Design review of the part built by this model. Coordinates are the model's own, in mm. Face numbers are marked on the shaded views. A direction names the side the tool comes from. Coordinates: 2 decimals unless noted, no trailing zeros. Order: outer loops, then holes, each group sorted by start corner. A loop starts at its lowest first (then second) coordinate and runs counter-clockwise, first axis right, second up. Notation, with made-up numbers: (77.25, 34.25) -> (124.25, 34.25) arc R12 ccw to (124.25, 50.25) -> close; hole circle Ø8 at (31.25, 17.5). An arc over 180 degrees is marked (long way). Write item = value, one per line.
```python
from build123d import *

# Parameters (mm, degrees)
SALIENTE_EXTRUIR1_DEPTH = 8
CROQUIS2_R              = 4.875
SALIENTE_EXTRUIR2_DEPTH = 28
MATRIZL1_COUNT          = 2
MATRIZL1_PITCH          = 25
MATRIZL1_COUNT_DIR2     = 2
MATRIZL1_PITCH_DIR2     = 25
CROQUIS3_R              = 2.65
CORTAR_EXTRUIR1_DEPTH   = 5.3
CROQUIS4_W              = 9.313425885
CROQUIS4_H              = 1.82271115
CROQUIS4_H_2            = 1.039944003
CROQUIS4_W_2            = 1.041549228
CROQUIS4_H_3            = 6.922662644
CROQUIS4_H_4            = 1.224371708
CORTAR_EXTRUIR2_DEPTH   = 2.5


with BuildPart() as part:
    # Croquis1 → Saliente-Extruir1 (new body)
    with BuildSketch(Plane(origin=(0, 0, 0), x_dir=(1, 0, 0), z_dir=(0, 1, 0))):
        with BuildLine():
            Line((-14.479225386, 25.911355575), (15.520774614, 25.911355575))
            ThreePointArc((15.520774614, 25.911355575), (22.591842426, 22.982423386), (25.520774614, 15.911355575))
            Line((25.520774614, 15.911355575), (25.520774614, -14.088644425))
            ThreePointArc((25.520774614, -14.088644425), (22.591842426, -21.159712237), (15.520774614, -24.088644425))
            Line((15.520774614, -24.088644425), (-14.479225386, -24.088644425))
            ThreePointArc((-14.479225386, -24.088644425), (-21.550293198, -21.159712237), (-24.479225386, -14.088644425))
            Line((-24.479225386, -14.088644425), (-24.479225386, 15.911355575))
            ThreePointArc((-24.479225386, 15.911355575), (-21.550293198, 22.982423386), (-14.479225386, 25.911355575))
        make_face()
    extrude(amount=SALIENTE_EXTRUIR1_DEPTH)

    # Croquis2 → Saliente-Extruir2 (add)
    with BuildSketch(Plane(origin=(0, 8, 0), x_dir=(1, 0, 0), z_dir=(0, 1, 0))):
        with Locations(Location((-11.979225386, 13.411355575, 0), (0, 0, 270))):
            Circle(CROQUIS2_R)
    saliente_extruir2 = extrude(amount=SALIENTE_EXTRUIR2_DEPTH)

    # MatrizL1: Saliente-Extruir2 2 × 2
    with Locations(*[(i * MATRIZL1_PITCH, 0, j * MATRIZL1_PITCH_DIR2) for i in range(MATRIZL1_COUNT) for j in range(MATRIZL1_COUNT_DIR2) if (i, j) != (0, 0)]):
        add(saliente_extruir2)

    # Croquis3 → Cortar-Extruir1 (cut)
    with BuildSketch(Plane(origin=(0, 8, 0), x_dir=(1, 0, 0), z_dir=(0, 1, 0))):
        with Locations(Location((0.520774614, 0.911355575, 0), (0, 0, 270))):
            Circle(CROQUIS3_R)
        with Locations(Location((0.520774614, 21.411355575, 0), (0, 0, 270))):
            Circle(CROQUIS3_R)
        with Locations(Location((0.520774614, -19.588644425, 0), (0, 0, 270))):
            Circle(CROQUIS3_R)
        with Locations(Location((-19.979225386, 0.911355575, 0), (0, 0, 270))):
            Circle(CROQUIS3_R)
        with Locations(Location((21.020774614, 0.911355575, 0), (0, 0, 270))):
            Circle(CROQUIS3_R)
    extrude(amount=-CORTAR_EXTRUIR1_DEPTH, mode=Mode.SUBTRACT)

    # Croquis4 → Cortar-Extruir2 (cut)
    with BuildSketch(Plane(origin=(0, 8, 0), x_dir=(1, 0, 0), z_dir=(0, 1, 0))):
        with Locations((0.889291465, -25)):
            Rectangle(CROQUIS4_W, CROQUIS4_H)
        with Locations((0.889291465, -23.568672424)):
            Rectangle(CROQUIS4_W, CROQUIS4_H_2)
        with Locations((25, 0.799054751)):
            Rectangle(CROQUIS4_W_2, CROQUIS4_H_3)
        with Locations((0.889291465, 25.299169721)):
            Rectangle(CROQUIS4_W, CROQUIS4_H_4)
        Polygon((-26.668299848, 4.260386073), (-26.668299848, -2.662276571), (-24.479225386, -2.662276571), (-23.262085841, -2.662276571), (-23.262085841, 4.260386073), (-24.479225386, 4.260386073), align=None)
    extrude(amount=-CORTAR_EXTRUIR2_DEPTH, mode=Mode.SUBTRACT)


solid = part.part
```
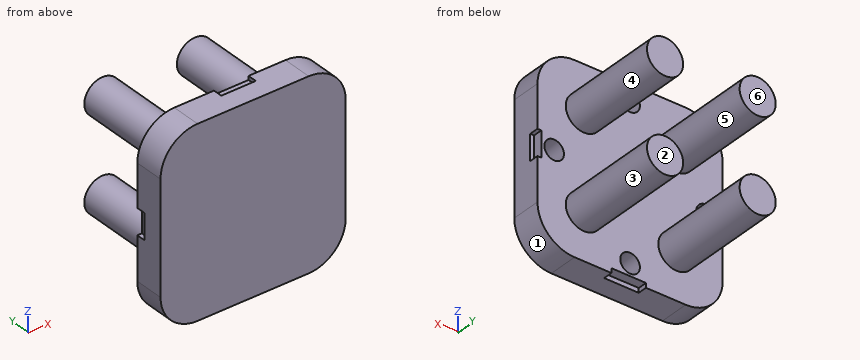
(1) For L1, parallel to Y at x = 18, z = 12; L2, parallel to X at y = 12, z = -13; L3, parallel to X at y = 29, z = -16, list the stretches that pass through material, from the lowest coordinate up.
Report:
L1 = 0 to 8
L2 = -16.84 to -7.12, 8.16 to 17.88
L3 = -16.11 to -7.85, 8.89 to 17.15
(2) We need section A-A (z = 15.5). Write out the cut boundary in (x, y), and give its area (3 significant figures).
Report:
outline = (-24.38, 0) -> (25.42, 0) -> (25.42, 8) -> (15.93, 8) -> (15.93, 36) -> (10.11, 36) -> (10.11, 8) -> (-9.07, 8) -> (-9.07, 36) -> (-14.89, 36) -> (-14.89, 8) -> (-24.38, 8) -> close
area = 724 mm²
(3) Insertion check: pin 1 (1.6 mm diameter, centred on x = 1.5, z = -0.5, fed in from +Y); pin 2 (8 mm diameter, centred on x = 19.5, y = 18, fed in from +Z); pin 3 (0.8 mm diameter, centred on x = 1, y = 7, fed in from -Z); pin 4 (10 mm diameter, centred on x = -7, z = 10.5, fed in from -Y). Each pin has a flat end and moves straight along its axis. Give the tip position at first contact, or say it passes through.
Report:
pin_1 = 2.7
pin_2 = 15.79
pin_3 = -24.69
pin_4 = 0
(4) We need section B-B (x = -18). Write out the cut boundary in (y, z), and give its area (3 significant figures).
Report:
outline = (0, -25.27) -> (8, -25.27) -> (8, -2.67) -> (2.7, -2.67) -> (2.7, 0.85) -> (8, 0.85) -> (8, 23.45) -> (0, 23.45) -> close
area = 371 mm²
(5) We need section D-D (y = 15.5). Write out the cut boundary in (x, z) (3 decimals).
Report:
outline = circle Ø9.75 at (-11.979, -13.411); circle Ø9.75 at (-11.979, 11.589); circle Ø9.75 at (13.021, -13.411); circle Ø9.75 at (13.021, 11.589)
(6) For the marked faces 5 and 6, list the 3-axis set-ups (+Z, -Z, +X, -X, +Y, -Y) from which the entire face can be reached by the end or side of a thin tool; tool diameter is ignored.
Report:
face_5 = +Y
face_6 = +Z, -Z, +X, -X, +Y
(7) We need section C-C (y = 3.5). Write out the cut boundary in (x, z).
Report:
outline = (-24.48, -15.91) arc R10 ccw to (-14.48, -25.91) -> (15.52, -25.91) arc R10 ccw to (25.52, -15.91) -> (25.52, 14.09) arc R10 ccw to (15.52, 24.09) -> (-14.48, 24.09) arc R10 ccw to (-24.48, 14.09) -> close; hole circle Ø5.3 at (-19.98, -0.91); hole circle Ø5.3 at (0.52, -21.41); hole circle Ø5.3 at (0.52, -0.91); hole circle Ø5.3 at (0.52, 19.59); hole circle Ø5.3 at (21.02, -0.91)
(8) The part is to be moulded in two halves that separate along Z. For the marked faces 1, 2, 3 and 4, say which applies: released by +Z, released by -Z, zero draft, split by the parting line, or undercut.
Report:
face_1 = released by -Z
face_2 = zero draft
face_3 = undercut
face_4 = undercut
